from build123d import *
from OCP.BRepAlgoAPI import BRepAlgoAPI_Cut
from OCP.TopTools import TopTools_ListOfShape

# Parameters (mm, degrees)
SKETCH1_R           = 5
BOSS_EXTRUDE1_DEPTH = 12.7
FILLET1_R           = 2.54
SCALE1_SCALE        = 0.66
CUT_EXTRUDE1_DEPTH  = 91.122674321
FILLET2_R           = 2.54
CUT_EXTRUDE2_DEPTH  = 25.4


with BuildPart() as part:
    # Sketch1 → Boss-Extrude1 (new body)
    with BuildSketch(Plane(origin=(0, 0, 0), x_dir=(1, 0, 0), z_dir=(0, 1, 0))):
        with BuildLine():
            Line((-77.410829365, -8.41547619), (-13.284900793, -49.577415951))
            ThreePointArc((-13.284900793, -49.577415951), (-3.938658922, -50.351151369), (1.938436508, -43.042892142))
            Line((1.938436508, -43.042892142), (9.821507936, -1.880952381))
            ThreePointArc((9.821507936, -1.880952381), (7.707448469, 6.371439248), (0, 10))
            Line((0, 10), (-72.009, 10))
            Line((-72.009, 10), (-106.100184572, 10))
            Line((-106.100184572, 10), (-77.410829365, -8.41547619))
        make_face()
        with Locations(Location((0, 0, 0), (0, 0, 270))):
            Circle(SKETCH1_R, mode=Mode.SUBTRACT)
        with Locations(Location((-7.883071429, -41.161939761, 0), (0, 0, 270))):
            Circle(SKETCH1_R, mode=Mode.SUBTRACT)
    extrude(amount=BOSS_EXTRUDE1_DEPTH)

    # Fillet1
    fillet1_edges = [part.edges().sort_by_distance(p)[0] for p in [
        (-3.938658922, 12.7, 50.351151369),
        (5.879972222, 12.7, 22.461922261),
        (7.707448469, 12.7, -6.371439248),
        (-53.050092286, 12.7, -10),
        (-59.692542683, 12.7, 19.788707976),
        (-53.050092286, 0, -10),
        (7.707448469, 0, -6.371439248),
        (5.879972222, 0, 22.461922261),
        (-3.938658922, 0, 50.351151369),
        (-59.692542683, 0, 19.788707976),
    ]]
    fillet(fillet1_edges, radius=FILLET1_R)


with BuildPart() as part_1:
    # Scale1: scaled about (-33.401454618, 6.35, 11.856994793)
    add(part.part.scale(SCALE1_SCALE).moved(Location((-11.35649457, 2.159, 4.03137823))))


with BuildPart() as cut_extrude1_tool:
    # Sketch2 → Cut-Extrude1 (new, through all)
    with BuildSketch(Plane(origin=(0, 10.540994585, 0), x_dir=(1, 0, 0), z_dir=(0, 1, 0))):
        Polygon((-58.349296315, -4.187754758), (-23.578618247, -26.506785264), (-19.304220279, -4.187754758), align=None)
    extrude(amount=-CUT_EXTRUDE1_DEPTH)


with BuildPart() as part_2:
    add(part_1.part)

    # Cut-Extrude1: cut by cut_extrude1_tool, with a tolerance
    cut_extrude1_stock = TopTools_ListOfShape()
    cut_extrude1_stock.Append(part_2.part.wrapped)
    cut_extrude1_tools = TopTools_ListOfShape()
    cut_extrude1_tools.Append(cut_extrude1_tool.part.wrapped)
    cut_extrude1_cut = BRepAlgoAPI_Cut()
    cut_extrude1_cut.SetArguments(cut_extrude1_stock)
    cut_extrude1_cut.SetTools(cut_extrude1_tools)
    cut_extrude1_cut.SetFuzzyValue(0.00001)
    cut_extrude1_cut.Build()
    add(Compound.cast(cut_extrude1_cut.Shape()).solids(), mode=Mode.REPLACE)

    # Fillet2
    fillet2_edges = [part_2.edges().sort_by_distance(p)[0] for p in [
        (-58.349296315, 6.349997293, 4.187754758),
        (-19.304220279, 6.349997293, 4.187754758),
        (-23.578618247, 6.349997293, 26.506785264),
    ]]
    fillet(fillet2_edges, radius=FILLET2_R)

    # Sketch3 → Cut-Extrude2 (cut)
    with BuildSketch(Plane(origin=(-58.803077328, 0, -37.745242535), x_dir=(0, -1, 0), z_dir=(-0.841547619047619, 0, -0.5401829364902999))):
        Polygon((-5.714994585, 41.799889271), (-5.714994585, 39.894889271), (-5.079994585, 39.894889271), (-5.079994585, 38.624889271), (-7.619994585, 38.624889271), (-7.619994585, 39.894889271), (-6.984994585, 39.894889271), (-6.984994585, 41.799889271), align=None)
    extrude(amount=-CUT_EXTRUDE2_DEPTH, mode=Mode.SUBTRACT)


solid = part_2.part
Source: CAD feature listing. Evaluate the final solid. Frame: model axes, mm. A direction names the side the tool comes from. Give positions to 0.01 mm unless a question says otherwise; leave off trailing zeros. Write each loop counter-clockwise with the first axis right and the second up, starting at its lowest first coordinate (ties: lowest second). Pieces come first, ordered by that corner, then holes. Notation, with made-up numbers: (27, -39) - (52, -39) arc R20 cw to (52, -11) - close; hole circle Ø1 at (-3.5, -14.5). An arc over 180 degrees is marked (long way). Write item = value, one per line. Start each with the question number.
Q1. Pin query (flat end, axial travel): pin 1 Ø4 at (x, y) = (-39, 4.5) entering from +Z; pin 2 Ø5 at (y, z) = (5, 6) entering from -X; pin 3 Ø1.5 at (x, y) = (-27, 4.5) entering from +Z. Return the tip coordinate at first contact, or that it passes through.
Q2. Draft query along Z for faces 4 (the flat face through (-46, 6, -2.569)), 5 (the flat face through (-34, 2.159, 4)), 6 (the cylindrical face through (-13.287, 6.291, 30.769)). Return one class per face: +Z half, -Z half, draft (parallel to the pull), parting line (faces both ways), or undercut.
Q3. Reachability of faces 1 (the flat face through (-67.02, 6.33, 2.88)), 2 (the cylindrical face through (-7.91, 2.66, 18.58)), 3 (the flat face through (-36, 6, 4.188)) from +Z, -Z, +X, -X, +Y, -Y: full face, straight path, thin tool, end or side. Return the list, or none.
Q4. Cut plane A-A, the plane y = 3. Return loops of the section in (x, z), then the cut area to 3 significant figures.
Q5. Material intervals for probe 1 along X at (y, z) = (6.5, 5); probe 2 along Z at (x, y) = (-14, 7.5); probe 3 along Z at (x, y) = (-28, 7.25), sorted ascending.
Computed values:
q1.pin_1 = 25.92
q1.pin_2 = -71.93
q1.pin_3 = 32.82
q2.face_4 = -Z half
q2.face_5 = draft
q2.face_6 = undercut
q3.face_1 = none
q3.face_2 = +Z, +X, -Y
q3.face_3 = +Y, -Y
q4.outline = (-80.62, -2.35) - (-11.36, -2.35) arc R6.38 ccw to (-5.09, 5.23) - (-10.3, 32.4) arc R6.38 ccw to (-20, 36.56) - close; hole (-51.06, 8.87) arc R2.54 ccw to (-49.69, 4.19) - (-22.38, 4.19) arc R2.54 ccw to (-19.88, 7.21) - (-22.87, 22.82) arc R2.54 ccw to (-26.74, 24.48) - close; hole circle Ø6.6 at (-16.56, 31.2); hole circle Ø6.6 at (-11.36, 4.03)
q4.area = 1,170 mm²
q5.probe_1 = -63.71 to -51.55, -20.51 to -14.51, -8.2 to -4.83
q5.probe_2 = -2.57 to 2.06, 6.01 to 29.12, 33.28 to 37.28
q5.probe_3 = -2.57 to 4.19, 23.67 to 31.7
